```python
from build123d import *

# Parameters (mm, degrees)
CROQUIS2_W              = 30
CROQUIS2_H              = 17.375045376
SALIENTE_EXTRUIR1_DEPTH = 2
CROQUIS3_R              = 4
SALIENTE_EXTRUIR2_DEPTH = 13


with BuildPart() as part:
    # Croquis2 → Saliente-Extruir1 (new body)
    with BuildSketch(Plane.XY):
        with Locations((0, -3.687522688)):
            Rectangle(CROQUIS2_W, CROQUIS2_H)
    extrude(amount=SALIENTE_EXTRUIR1_DEPTH)

    # Croquis3 → Saliente-Extruir2 (add)
    with BuildSketch(Plane.XY.offset(2)):
        Circle(CROQUIS3_R)
        with BuildLine():
            Line((-15, 5), (-14.271293534, 5))
            ThreePointArc((-14.271293534, 5), (-9.727126272, 3.291298824), (-7.434621256, -0.98813298))
            ThreePointArc((-7.434621256, -0.98813298), (0, -7.5), (7.434621256, -0.98813298))
            ThreePointArc((7.434621256, -0.98813298), (9.727126272, 3.291298824), (14.271293534, 5))
            Line((14.271293534, 5), (15, 5))
            Line((15, 5), (15, -12.375045376))
            Line((15, -12.375045376), (-15, -12.375045376))
            Line((-15, -12.375045376), (-15, 5))
        make_face()
    extrude(amount=SALIENTE_EXTRUIR2_DEPTH)


solid = part.part
```
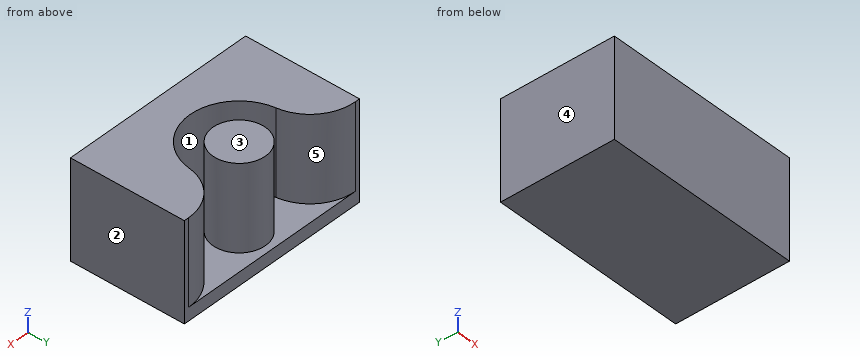
Can you work these out from the model? Positions are in its coordinate system, mm. Face numbers are marked on the shaded views. A direction names the side the tool comes from. Coordinates: 2 decimals unless noted, no trailing zeros. Write each loop counter-clockwise with the first axis right and the second up, starting at its lowest first coordinate (ties: lowest second). Pieces come first, ordered by that corner, then holes. Notation, with made-up numbers: M 59,14 L 79,14 A25 ccw 79,40 Z; hole C 47,77.5 d4. An arc over 180 degrees is marked long. Answer as CSV lines item,"result".
Item 1: Imagine slicing it at D-D on y = -4.5. List the corners of the cut face in (x, z) for me, plus the area to 3 significant figures.
Geometry results:
outline,"M -15,0 L 15,0 L 15,15 L 6,15 L 6,2 L -6,2 L -6,15 L -15,15 Z"
area,"294 mm2"
Item 2: Imagine slicing it at C-C on x = 0. List the corners of the cut face in (y, z) for me, plus the area to 3 significant figures.
Geometry results:
outline,"M -12.38,0 L 5,0 L 5,2 L 4,2 L 4,15 L -4,15 L -4,2 L -7.5,2 L -7.5,15 L -12.38,15 Z"
area,"202 mm2"
Item 3: Imagine slicing it at B-B on y = -2.5. List the corners of the cut face in (x, z) for me, plus the area to 3 significant figures.
Geometry results:
outline,"M -15,0 L 15,0 L 15,15 L 7.07,15 L 7.07,2 L 3.12,2 L 3.12,15 L -3.12,15 L -3.12,2 L -7.07,2 L -7.07,15 L -15,15 Z"
area,"347 mm2"
Item 4: Please list where these lines run through material, in increasing order: line 1 along X through (y, z) = (-2.5, 9.5); line 2 along X through (y, z) = (-2.75, 9.25); line 3 along Z through (x, y) = (2.75, -5).
Geometry results:
line 1,"x = -15 to -7.07, -3.12 to 3.12, 7.07 to 15"
line 2,"x = -15 to -6.98, -2.9 to 2.9, 6.98 to 15"
line 3,"z = 0 to 2"
Item 5: We'd pull the mould along X, two halves only. Please class the marked faces 3, 4 and 5: +X half, -X half, draft (parallel to the pull), parting line (faces both ways), or undercut.
Geometry results:
face 3,"draft"
face 4,"-X half"
face 5,"undercut"
Item 6: Imagine slicing it at A-A on z = 10.5. List the corners of the cut face in (x, y) for me.
Geometry results:
outline,"M -15,-12.38 L 15,-12.38 L 15,5 L 14.27,5 A6.9 ccw 7.43,-0.99 A7.5 cw -7.43,-0.99 A6.9 ccw -14.27,5 L -15,5 Z; C 0,0 d8"
Item 7: On a 3-axis mill with a long thin cutter (end or side, diameter ignored), from which of +Z, -Z, +X, -X, +Y, -Y can I reach the whole of each face in a straight line? I mean the marked faces 1 and 2. Say none if no direction works.
Geometry results:
face 1,"+Z"
face 2,"+Z, -Z, +X, +Y, -Y"
Item 8: I'm going to push flat-ended pins straight in: P1, Ø6, axis at x = -5.5, y = 0, coming from the +Z side; P2, Ø6, axis at x = 8.5, z = 5.5, coming from the +Y side; P3, Ø1.5, axis at x = 12, z = 12, coming from the +Y side. Where does each tip first touch, or does it pass through?
Geometry results:
P1,"stops at z = 15"
P2,"stops at y = 4.42"
P3,"stops at y = 4.83"
